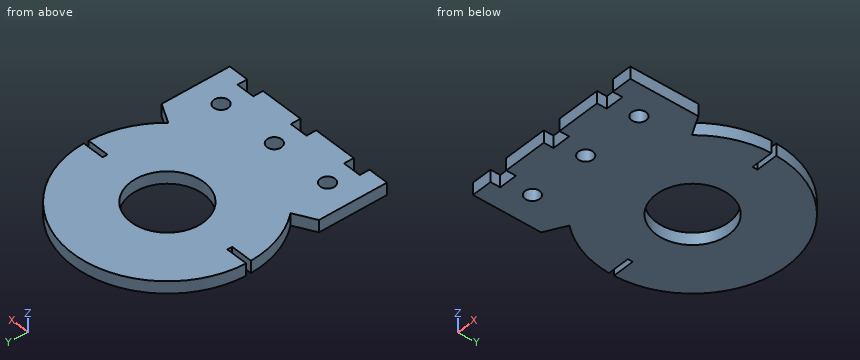
```python
from build123d import *

# Parameters (mm, degrees)
SKETCH1_R           = 0.6
SKETCH1_R_2         = 3
BOSS_EXTRUDE1_DEPTH = 0.5


with BuildPart() as part:
    # Sketch1 → Boss-Extrude1 (new, symmetric)
    with BuildSketch(Plane.XY):
        with BuildLine():
            Line((-7.5, -6), (-5.835451996, -5.1))
            ThreePointArc((-5.835451996, -5.1), (-7.219840415, -2.81716247), (-7.747418925, -0.2))
            Line((-7.747418925, -0.2), (-5.947418925, -0.2))
            Line((-5.947418925, -0.2), (-5.947418925, 0))
            Line((-5.947418925, 0), (-5.947418925, 0.2))
            Line((-5.947418925, 0.2), (-7.747418925, 0.2))
            ThreePointArc((-7.747418925, 0.2), (0, 7.75), (7.747418925, 0.2))
            Line((7.747418925, 0.2), (5.947418925, 0.2))
            Line((5.947418925, 0.2), (5.947418925, 0))
            Line((5.947418925, 0), (5.947418925, -0.2))
            Line((5.947418925, -0.2), (7.747418925, -0.2))
            ThreePointArc((7.747418925, -0.2), (7.219840415, -2.81716247), (5.835451996, -5.1))
            Line((5.835451996, -5.1), (7.5, -6))
            Line((7.5, -6), (7.5, -11.6))
            Line((7.5, -11.6), (5.83, -11.6))
            Line((5.83, -11.6), (5.83, -10.8))
            Line((5.83, -10.8), (4.33, -10.8))
            Line((4.33, -10.8), (4.33, -11.6))
            Line((4.33, -11.6), (0.75, -11.6))
            Line((0.75, -11.6), (0.75, -10.8))
            Line((0.75, -10.8), (-0.75, -10.8))
            Line((-0.75, -10.8), (-0.75, -11.6))
            Line((-0.75, -11.6), (-4.33, -11.6))
            Line((-4.33, -11.6), (-4.33, -10.8))
            Line((-4.33, -10.8), (-5.83, -10.8))
            Line((-5.83, -10.8), (-5.83, -11.6))
            Line((-5.83, -11.6), (-7.5, -11.6))
            Line((-7.5, -11.6), (-7.5, -6))
        make_face()
        with Locations((-5.08, -8.8)):
            Circle(SKETCH1_R, mode=Mode.SUBTRACT)
        with Locations((0, -8.8)):
            Circle(SKETCH1_R, mode=Mode.SUBTRACT)
        with Locations((5.08, -8.8)):
            Circle(SKETCH1_R, mode=Mode.SUBTRACT)
        Circle(SKETCH1_R_2, mode=Mode.SUBTRACT)
    extrude(amount=BOSS_EXTRUDE1_DEPTH, both=True)


solid = part.part
```
CAD build for the part. Positions are in the model's coordinates, mm. Round coordinates to 2 decimals unless told otherwise and drop trailing zeros. Loops run counter-clockwise (first coordinate to the right, second up) from the corner with the lowest first, then second, coordinate; pieces in that order, holes last. Notation, with made-up numbers: M 81.25,47 L 129.25,47 A34 cw 129.25,82 Z; hole C -24.5,51.5 d6. An arc over 180 degrees is marked long. Use a Markdown table: item, result. Add a question column.
(1) Flat gauge pin, fed straight in: pin 1 (0.6 mm diameter, centred on y = -11, z = 0, fed in from +X). Where does the tip first touch, or does it go through?
(2) Cut at D-D (x = -5.08). Give the cut face in (y, z).
(3) Cut at B-B (y = -8.8). Give the cut face in (x, z).
(4) Cut at A-A (z = 0.05). State how many separate pieces and enclosed holes the cut face has, and give its area (3 significant figures).
(5) Drill centre lines: line 1 (Y direction, x = 0, z = 0.2); line 2 (X direction, y = -8.75, z = -0.1); line 3 (Y direction, x = 7, z = 0.45). Where is each one in solid material? Low to high.
(6) Cut at C-C (x = 0). Give the cut face in (y, z), and give its area (4 significant figures).
Geometry says:
| question | item | result |
|---|---|---|
| 1 | pin 1 | stops at x = 7.5 |
| 2 | outline | M -10.8,-0.5 L -9.4,-0.5 L -9.4,0.5 L -10.8,0.5 Z; M -8.2,-0.5 L 5.85,-0.5 L 5.85,0.5 L -8.2,0.5 Z |
| 3 | outline | M -7.5,-0.5 L -5.68,-0.5 L -5.68,0.5 L -7.5,0.5 Z; M -4.48,-0.5 L -0.6,-0.5 L -0.6,0.5 L -4.48,0.5 Z; M 0.6,-0.5 L 4.48,-0.5 L 4.48,0.5 L 0.6,0.5 Z; M 5.68,-0.5 L 7.5,-0.5 L 7.5,0.5 L 5.68,0.5 Z |
| 4 | separate pieces | 1 |
| 4 | enclosed holes | 4 |
| 4 | area | 227 mm² |
| 5 | line 1 | y = -10.8 to -9.4, -8.2 to -3, 3 to 7.75 |
| 5 | line 2 | x = -7.5 to -5.68, -4.48 to -0.6, 0.6 to 4.48, 5.68 to 7.5 |
| 5 | line 3 | y = -11.6 to -5.73, -3.33 to -0.2, 0.2 to 3.33 |
| 6 | outline | M -10.8,-0.5 L -9.4,-0.5 L -9.4,0.5 L -10.8,0.5 Z; M -8.2,-0.5 L -3,-0.5 L -3,0.5 L -8.2,0.5 Z; M 3,-0.5 L 7.75,-0.5 L 7.75,0.5 L 3,0.5 Z |
| 6 | area | 11.35 mm² |
